```python
from build123d import *

# Parameters (mm, degrees)
F0_W     = 88.9
F0_H     = 6.35
F1_DEPTH = 3.175
F2_R     = 4.7625
F3_DEPTH = 3.175
F4_R     = 4.7625
F5_DEPTH = 3.175
F6_R     = 2.024984
F6_R_2   = 1.6256
F7_DEPTH = 3.175


with BuildPart() as f1:
    # F0 (on Right) → F1 (new body)
    with BuildSketch(Plane.YZ):
        with Locations((-10.188125, 17.503159)):
            Rectangle(F0_W, F0_H)
    extrude(amount=F1_DEPTH)

    # F2 (on Right) → F3 (join)
    with BuildSketch(Plane.YZ):
        with Locations((-54.662056, 17.522926)):
            Circle(F2_R)
    extrude(amount=F3_DEPTH)

    # F4 (on Right) → F5 (join)
    with BuildSketch(Plane.YZ):
        with Locations((34.302156, 17.490556)):
            Circle(F4_R)
    extrude(amount=F5_DEPTH)

    # F6 (on face) → F7 (cut)
    with BuildSketch(Plane.YZ.offset(3.175)):
        with Locations((-54.662056, 17.522926)):
            Circle(F6_R)
        with Locations((34.302156, 17.490556)):
            Circle(F6_R_2)
    extrude(amount=-F7_DEPTH, mode=Mode.SUBTRACT)


solid = f1.part
```
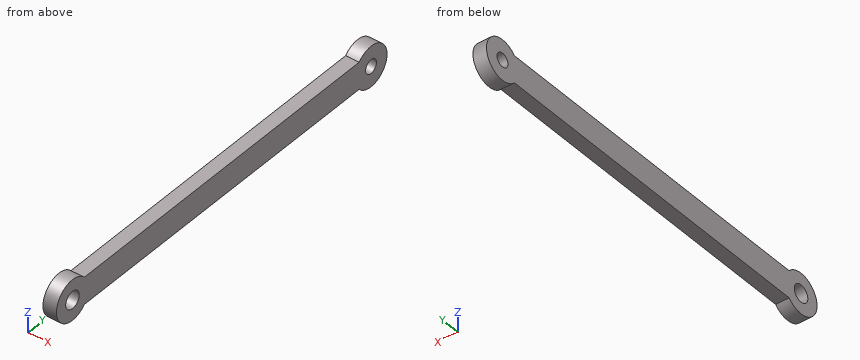
Work out the finished part from the listing and answer in its coordinate system (mm). Give positions to 0.01 mm unless a question says otherwise; leave off trailing zeros. Loops run counter-clockwise (first coordinate to the right, second up) from the corner with the lowest first, then second, coordinate; pieces in that order, holes last. Notation, with made-up numbers: (81, -31.5) -> (106, -31.5) arc R16 ccw to (106, -9.5) -> close; hole circle Ø9 at (21.25, 88). An arc over 180 degrees is marked (long way). Put each result on its own line as item: value. Start each with the question number.
Item 1: Find the intervals of material crossed by L1, parallel to Y at x = 1.5, z = 17; L2, parallel to Y at x = 2, z = 17.75; L3, parallel to Z at x = 2.95, y = -10, in increasing order. Write a range as [from, to].
Item 2: The part is cut by section A-A (y = -22). Give the vertices of the cut face in (x, z) (3 decimals).
Item 3: Each of these flat-tipped pins is pushed along its axis until it touches: P1, Ø2, axis at y = 34.3, z = 17.49, coming from the +X side; P2, Ø1, axis at x = 1.5, y = 5.5, coming from the -Z side. Where does it stop, or does it pass through?
Item 4: The part is cut by section B-B (x = 1.7). Give the vertices of the cut face in (y, z) (1 decimal).
Answers below:
1. L1: [-59.4, -56.62], [-52.71, 32.75], [35.85, 39.04]
1. L2: [-59.42, -56.67], [-52.65, 32.7], [35.91, 39.06]
1. L3: [14.33, 20.68]
2. outline: (0, 14.328) -> (3.175, 14.328) -> (3.175, 20.678) -> (0, 20.678) -> close
3. P1: through
3. P2: z = 14.33
4. outline: (-51.1, 14.3) -> (30.7, 14.3) arc R4.8 ccw (long way) to (30.8, 20.7) -> (-51.1, 20.7) arc R4.8 ccw (long way) to start; hole circle Ø4 at (-54.7, 17.5); hole circle Ø3.3 at (34.3, 17.5)
